Autodesk Inventor part; units mm, degrees
ref_plane "YZ Plane" through (0, 0, 0) normal (1, 0, 0) x (0, 1, 0)
ref_plane "XZ Plane" through (0, 0, 0) normal (0, 1, 0) x (-1, 0, 0)
ref_plane "XY Plane" through (0, 0, 0) normal (0, 0, 1) x (1, 0, 0)
sketch "Sketch1" plane through (0, 0, 0) normal (0, 0, 1) x (1, 0, 0)
  line L0 (9.893, 6.4872) -> (9.893, 9.4872)
  line L1 (31.893, 6.4872) -> (31.893, 9.4872)
  arc A0 (44.393, 68.4872) -> (22.393, 68.4872) centre (33.393, 68.4872) ccw
  line L2 (9.893, 6.4872) -> (31.893, 6.4872)
  line L3 (9.893, 9.4872) -> (22.393, 31.1378)
  line L4 (9.893, 9.4872) -> (39.4953, 9.4872) construction
  line L5 (31.893, 9.4872) -> (44.393, 31.1378)
  line L6 (44.393, 68.4872) -> (44.393, 31.1378)
  line L7 (22.393, 68.4872) -> (22.393, 31.1378)
  circle A1 centre (33.393, 68.4872) radius 4.5
  point P0 (0, 0)
  dimension "d0" = 62
  dimension "d1" = 1.5
  dimension "d2" = 3
  dimension "d3" = 3
  dimension "d5" = 22
  dimension "d6" = 60
  dimension "d7" = 22
  dimension "d8" = 9
extrude "Extrusion1" add sketch "Sketch1" along normal blind 47
sketch "Sketch2" plane through (9.893, 6.4872, 0) normal (-1, 0, 0) x (0, 0, 1)
  line L0 (0, 3) -> (47, 3)
  line L1 (0, 73) -> (47, 73)
  line L2 (3, 3) -> (3, 73)
  line L3 (3, 73) -> (44, 73)
  line L4 (44, 73) -> (44, 3)
  line L5 (0, 3) -> (0, 24.6506)
  line L6 (47, 24.6506) -> (47, 62)
  line L7 (3, 3) -> (44, 3)
  point P0 (0, -6.4872)
  dimension "d11" = 3
  dimension "d12" = 3
extrude "Extrusion2" cut sketch "Sketch2" against normal through all
sketch "Sketch3" plane through (9.893, 6.4872, 0) normal (0, -1, 0) x (1, 0, 0)
  circle A0 centre (11, 23.5) radius 4.5
  line L0 (22, 0) -> (0, 0)
  point P0 (-9.893, 0)
  dimension "d15" = 9
  dimension "d18" = 23.5
extrude "Extrusion3" cut sketch "Sketch3" against normal through all
sketch "Sketch4" plane through (0, 0, 47) normal (0, 0, 1) x (1, 0, 0)
  circle A0 centre (33.393, 38.4872) radius 4.5
  circle A1 centre (33.393, 46.9872) radius 1
  circle A2 centre (27.3825, 44.4976) radius 1
  circle A3 centre (24.893, 38.4872) radius 1
  circle A4 centre (27.3825, 32.4768) radius 1
  circle A5 centre (33.393, 29.9872) radius 1
  circle A6 centre (39.4034, 32.4768) radius 1
  circle A7 centre (41.893, 38.4872) radius 1
  circle A8 centre (39.4034, 44.4976) radius 1
  point P0 (0, 0)
extrude "Extrusion4" cut sketch "Sketch4" against normal through all contours A1 | A2 | A3 | A4 | A5 | A6 | A7 | A8
sketch "Sketch5" plane through (9.893, 9.4872, 44) normal (0, 1, 0) x (1, 0, 0)
  circle A0 centre (11, 20.5) radius 4.5
  circle A1 centre (11, 29) radius 1
  circle A2 centre (4.9896, 26.5104) radius 1
  circle A3 centre (2.5, 20.5) radius 1
  circle A4 centre (4.9896, 14.4896) radius 1
  circle A5 centre (11, 12) radius 1
  circle A6 centre (17.0104, 14.4896) radius 1
  circle A7 centre (19.5, 20.5) radius 1
  circle A8 centre (17.0104, 26.5104) radius 1
  point P0 (-9.893, 44)
extrude "Extrusion5" cut sketch "Sketch5" against normal through all contours A1 | A2 | A3 | A4 | A5 | A6 | A7 | A8
properties part number "Neck" material "Aluminum-6061"
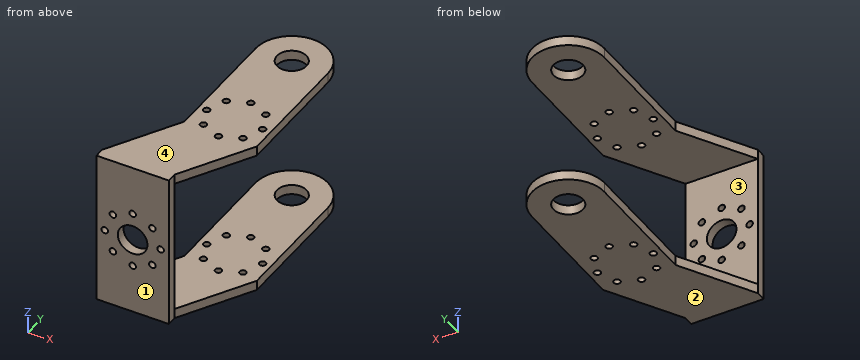
Build history of the part. All positions in model axes, mm. Face numbers are marked on the shaded views. Give positions to 0.01 mm unless a question says otherwise; leave off trailing zeros. Order: outer loops, then holes, each group sorted by start corner. A loop starts at its lowest first (then second) coordinate and runs counter-clockwise, first axis right, second up. Notation, with made-up numbers: M 39.25,37.25 L 49.25,37.25 A20 ccw 49.25,54.25 Z; hole C 23,-7 d11. An arc over 180 degrees is marked long. Return JSON: item names as keys, results as strings.
Q1. Band-saw the part on A-A (z = 15). Give the cut face in (x, y).
Answer list:
{"outline": "M 9.89,6.49 L 19.89,6.49 L 19.89,9.49 L 9.89,9.49 Z; M 21.89,6.49 L 31.89,6.49 L 31.89,9.49 L 21.89,9.49 Z"}
Q2. Two-plate mould, pull along Z, no slides. Class the marked faces 1, 2, 3 and 4: pulls with the +Z half, pulls with the -Z half, needs draft (parallel to the pull), parting line crosses it, or undercut.
Answer list:
{"face 1": "needs draft", "face 2": "pulls with the -Z half", "face 3": "undercut", "face 4": "pulls with the +Z half"}
Q3. Band-saw the part on B-B (z = 23.5). Give the cut face in (x, y).
Answer list:
{"outline": "M 9.89,6.49 L 11.39,6.49 L 11.39,9.49 L 9.89,9.49 Z; M 13.39,6.49 L 16.39,6.49 L 16.39,9.49 L 13.39,9.49 Z; M 25.39,6.49 L 28.39,6.49 L 28.39,9.49 L 25.39,9.49 Z; M 30.39,6.49 L 31.89,6.49 L 31.89,9.49 L 30.39,9.49 Z"}
Q4. Flat gauge pins, fed straight in: pin 1 (12 mm diameter, centred on x = 30.5, z = 14, fed in from +Y); pin 2 (2.5 mm diameter, centred on y = 8.5, z = 28.5, fed in from +X). Where does each tip first touch, or does it go through?
Answer list:
{"pin 1": "stops at y = 9.49", "pin 2": "stops at x = 31.89"}
Q5. Wall check: probe 1 along Z at (x, y) = (30.5, 47.5); probe 2 along Y at (x, z) = (22.5, 10.5); probe 3 along Y at (x, z) = (20.5, 2). Give the ranges that are in metal, low to high. Write a range as from..to.
Answer list:
{"probe 1": "z = 0..3, 44..47", "probe 2": "y = 6.49..9.49", "probe 3": "y = 6.49..27.86"}
Q6. Band-saw the part on D-D (y = 72). Give the cut face in (x, z).
Answer list:
{"outline": "M 22.97,0 L 30.58,0 L 30.58,3 L 22.97,3 Z; M 22.97,44 L 30.58,44 L 30.58,47 L 22.97,47 Z; M 36.21,0 L 43.82,0 L 43.82,3 L 36.21,3 Z; M 36.21,44 L 43.82,44 L 43.82,47 L 36.21,47 Z"}
Q7. Band-saw the part on C-C (y = 21). Give the cut face in (x, z).
Answer list:
{"outline": "M 16.54,0 L 38.54,0 L 38.54,3 L 16.54,3 Z; M 16.54,44 L 38.54,44 L 38.54,47 L 16.54,47 Z"}
